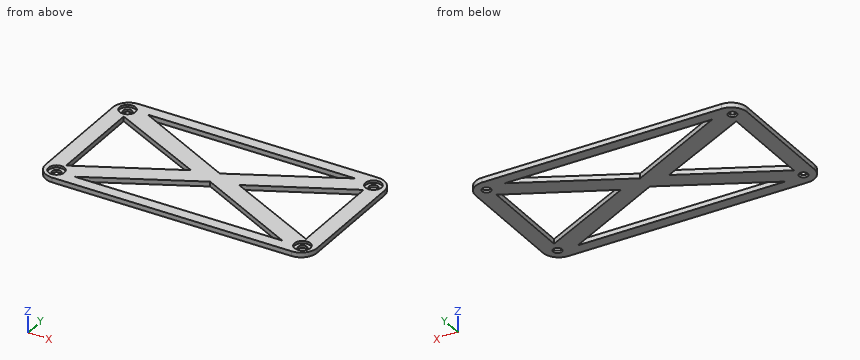
from build123d import *

# Parameters (mm, degrees)
EXTRUDE_1_DEPTH          = 3
CUT_EXTRUDE_1_DEPTH      = 39
CUT_EXTRUDE_1_DEPTH_BACK = 10
SKETCH_2_R               = 2.75
SKETCH_3_R               = 5
CUT_EXTRUDE_2_DEPTH      = 1.5


with BuildPart() as part:
    # 草图1 → 凸台-拉伸1 (new body)
    with BuildSketch(Plane.XY):
        with BuildLine():
            Line((-72.574116531, 45.487390308), (77.425883469, 45.487390308))
            ThreePointArc((77.425883469, 45.487390308), (84.496951281, 42.558458119), (87.425883469, 35.487390308))
            Line((87.425883469, 35.487390308), (87.425883469, -34.512609692))
            ThreePointArc((87.425883469, -34.512609692), (84.496951281, -41.583677504), (77.425883469, -44.512609692))
            Line((77.425883469, -44.512609692), (-72.574116531, -44.512609692))
            ThreePointArc((-72.574116531, -44.512609692), (-79.645184343, -41.583677504), (-82.574116531, -34.512609692))
            Line((-82.574116531, -34.512609692), (-82.574116531, 35.487390308))
            ThreePointArc((-82.574116531, 35.487390308), (-79.645184343, 42.558458119), (-72.574116531, 45.487390308))
        make_face()
    extrude(amount=EXTRUDE_1_DEPTH)

    # 草图2 → 切除-拉伸1 (cut, two sides: drawn at the far end of the back side and taken through both)
    with BuildSketch(Plane.XY.offset(3).offset(-CUT_EXTRUDE_1_DEPTH_BACK)):
        with Locations((-74.574116531, 37.487390308)):
            Circle(SKETCH_2_R)
        with Locations((-74.574116531, -36.512609692)):
            Circle(SKETCH_2_R)
        with Locations((79.425883469, 37.487390308)):
            Circle(SKETCH_2_R)
        with Locations((79.425883469, -36.512609692)):
            Circle(SKETCH_2_R)
        Polygon((-62.574116531, 38.487390308), (2.425883469, 5.487390308), (67.425883469, 38.487390308), align=None)
        Polygon((-72.574116531, 30.156085606), (-12.574116531, 0.487390308), (-72.574116531, -29.843914394), align=None)
        Polygon((2.425883469, -4.512609692), (-62.574116531, -37.512609692), (67.425883469, -37.512609692), align=None)
        Polygon((17.425883469, 0.487390308), (77.425883469, 30.487390308), (77.425883469, -29.512609692), align=None)
    extrude(amount=CUT_EXTRUDE_1_DEPTH + CUT_EXTRUDE_1_DEPTH_BACK, mode=Mode.SUBTRACT)

    # 草图3 → 切除-拉伸2 (cut)
    with BuildSketch(Plane.XY.offset(3)):
        with Locations((-74.574116531, 37.487390308)):
            Circle(SKETCH_3_R)
        with Locations((79.425883469, 37.487390308)):
            Circle(SKETCH_3_R)
        with Locations((79.425883469, -36.512609692)):
            Circle(SKETCH_3_R)
        with Locations((-74.574116531, -36.512609692)):
            Circle(SKETCH_3_R)
    extrude(amount=-CUT_EXTRUDE_2_DEPTH, mode=Mode.SUBTRACT)


solid = part.part
For this review, take the finished solid that the model builds, in its own axes (mm). Round coordinates to 2 decimals unless told otherwise and drop trailing zeros. Write each loop counter-clockwise with the first axis right and the second up, starting at its lowest first coordinate (ties: lowest second). Pieces come first, ordered by that corner, then holes. Notation, with made-up numbers: (51, -38.5) - (87, -38.5) arc R24 cw to (87, -28.5) - close; hole circle Ø5 at (19.25, 42.5). An arc over 180 degrees is marked (long way). Use a Markdown table: item, result.
Q1. We need section C-C (x = 40). Give the boundary of the cut face in (y, z), plus the area to 3 significant figures.
Derived:
| item | result |
|---|---|
| outline | (-44.51, 0) - (-37.51, 0) - (-37.51, 3) - (-44.51, 3) - close; (-23.59, 0) - (-10.8, 0) - (-10.8, 3) - (-23.59, 3) - close; (11.77, 0) - (24.56, 0) - (24.56, 3) - (11.77, 3) - close; (38.49, 0) - (45.49, 0) - (45.49, 3) - (38.49, 3) - close |
| area | 119 mm2 |
Q2. We need section A-A (x = -1.5). Give the boundary of the cut face in (y, z).
Derived:
| item | result |
|---|---|
| outline | (-44.51, 0) - (-37.51, 0) - (-37.51, 3) - (-44.51, 3) - close; (-6.51, 0) - (7.48, 0) - (7.48, 3) - (-6.51, 3) - close; (38.49, 0) - (45.49, 0) - (45.49, 3) - (38.49, 3) - close |
Q3. Clearance check with flat-ended pins moving along their axes: pin 1 (4.5 mm diameter, centred on x = 79.43, y = -36.51, fed in from -Z); pin 2 (5 mm diameter, centred on x = -76, y = -35, fed in from +Z). State where each tip first meets the part, or that it passes through.
Derived:
| item | result |
|---|---|
| pin 1 | passes through |
| pin 2 | stops at z = 1.5 |
Q4. We need section B-B (y = -18). Give the boundary of the cut face in (x, z), plus the area to 3 significant figures.
Derived:
| item | result |
|---|---|
| outline | (-82.57, 0) - (-72.57, 0) - (-72.57, 3) - (-82.57, 3) - close; (-49.15, 0) - (-24.14, 0) - (-24.14, 3) - (-49.15, 3) - close; (28.99, 0) - (54.4, 0) - (54.4, 3) - (28.99, 3) - close; (77.43, 0) - (87.43, 0) - (87.43, 3) - (77.43, 3) - close |
| area | 211 mm2 |
Q5. Wall thickness on line 1 along X through (y, z) = (-39, 1.25); line 2 along X through (y, z) = (11, 0.4); line 3 along X through (y, z) = (-18, 1.4): over which ranges is each line inside the solid? List them lowest first.
Derived:
| item | result |
|---|---|
| line 1 | x = -81.51 to -75.75, -73.4 to 78.25, 80.6 to 86.36 |
| line 2 | x = -82.57 to -72.57, -33.83 to -8.43, 13.28 to 38.45, 77.43 to 87.43 |
| line 3 | x = -82.57 to -72.57, -49.15 to -24.14, 28.99 to 54.4, 77.43 to 87.43 |
Q6. We need section D-D (z = 2). State how many separate pieces and enclosed holes the cut face has, plus the area to 3 significant figures.
Derived:
| item | result |
|---|---|
| separate pieces | 1 |
| enclosed holes | 8 |
| area | 7,010 mm2 |
